Geometry check sheet. Reference: the model listing, model coordinates, mm. A direction names the side the tool comes from. Give positions to 0.01 mm unless a question says otherwise; leave off trailing zeros. Loops run counter-clockwise (first coordinate to the right, second up) from the corner with the lowest first, then second, coordinate; pieces in that order, holes last. Notation, with made-up numbers: (59.5, -20.75) -> (110.5, -20.75) arc R23 cw to (110.5, 15.25) -> close; hole circle Ø9 at (69, 53). An arc over 180 degrees is marked (long way). Answer as a JSON object with one key per item and string values.
from build123d import *

# Parameters (mm, degrees)
F1_DEPTH = 10
F2_R     = 3
F3_DEPTH = 10
F4_R     = 1.5
F5_DEPTH = 25
F6_R     = 3
F7_DEPTH = 5


with BuildPart() as f1:
    # F0 (on Right) → F1 (new body)
    with BuildSketch(Plane.YZ):
        Polygon((2.886751, 5), (-2.886751, 5), (-5.773503, 0), (-2.886751, -5), (2.886751, -5), (5.773503, 0), align=None)
    extrude(amount=F1_DEPTH)

    # F2 (on face) → F3 (join)
    with BuildSketch(Plane.YZ.offset(10)):
        Circle(F2_R)
    extrude(amount=F3_DEPTH)

    # F4 (on face) → F5 (cut)
    with BuildSketch(Plane(origin=(0, 0, 0), x_dir=(0, -1, 0), z_dir=(-1, 0, 0))):
        Circle(F4_R)
    extrude(amount=-F5_DEPTH, mode=Mode.SUBTRACT)

    # F6 (on face) → F7 (cut)
    with BuildSketch(Plane(origin=(0, 0, 0), x_dir=(0, -1, 0), z_dir=(-1, 0, 0))):
        Circle(F6_R)
    extrude(amount=-F7_DEPTH, mode=Mode.SUBTRACT)


solid = f1.part
1) Tool access check on faces 1 (the face through (15, -3, 0)), 2 (the face through (4.93, -4.35, -2.465)). Record the directions out of +Z, -Z, +X, -X, +Y, -Y that give a thin tool (end or side, any length) a straight path to the whole face; none if there is none.
Geometry check:
{"face 1": "+X", "face 2": "-Z, +X, -X, -Y"}
2) Section check D-D on x = 2. Record the cut outline in (y, z).
Geometry check:
{"outline": "(-5.77, 0) -> (-2.89, -5) -> (2.89, -5) -> (5.77, 0) -> (2.89, 5) -> (-2.89, 5) -> close; hole circle Ø6 at (0, 0)"}
3) Depth check by flat-ended pin: P1, Ø1.5, axis at y = 0, z = 2, coming from the -X side; P2, Ø5, axis at x = 15, z = 0, coming from the -Y side; P3, Ø1.5, axis at x = 2.5, y = -4, coming from the -Z side. Enter the tip coordinate at first touch or a pass-through.
Geometry check:
{"P1": "stops at x = 5", "P2": "stops at y = -3", "P3": "stops at z = -4.37"}
4) Material ranges on line 1 along Z through (x, y) = (3.5, 0); line 2 along Z through (x, y) = (14.5, 0); line 3 along X through (y, z) = (-4, -1.25), recorded low to high. Write a range as from..to.
Geometry check:
{"line 1": "z = -5..-3, 3..5", "line 2": "z = -3..-1.5, 1.5..3", "line 3": "x = 0..10"}
5) Section check B-B on x = 5.75. Record the cut outline in (y, z), plus the area to 3 significant figures.
Geometry check:
{"outline": "(-5.77, 0) -> (-2.89, -5) -> (2.89, -5) -> (5.77, 0) -> (2.89, 5) -> (-2.89, 5) -> close; hole circle Ø3 at (0, 0)", "area": "79.5 mm2"}
6) Section check C-C on z = -0.5. Record the cut outline in (x, y).
Geometry check:
{"outline": "(0, -5.48) -> (10, -5.48) -> (10, -2.96) -> (20, -2.96) -> (20, -1.41) -> (5, -1.41) -> (5, -2.96) -> (0, -2.96) -> close; (0, 2.96) -> (5, 2.96) -> (5, 1.41) -> (20, 1.41) -> (20, 2.96) -> (10, 2.96) -> (10, 5.48) -> (0, 5.48) -> close"}
7) Draft check along Y on faces 3 (the face through (5, -1.3, -1.3)), 4 (the face through (4.93, 4.35, 2.465)), 5 (the face through (4.93, -4.31, 2.535)), 6 (the face through (2, 3, 0)). Enter one of: pulls with the +Y half, pulls with the -Y half, needs draft (parallel to the pull), parting line crosses it, or undercut.
Geometry check:
{"face 3": "undercut", "face 4": "pulls with the +Y half", "face 5": "pulls with the -Y half", "face 6": "undercut"}
8) Section check A-A on y = 0. Record the cut outline in (x, z).
Geometry check:
{"outline": "(0, -5) -> (10, -5) -> (10, -3) -> (20, -3) -> (20, -1.5) -> (5, -1.5) -> (5, -3) -> (0, -3) -> close; (0, 3) -> (5, 3) -> (5, 1.5) -> (20, 1.5) -> (20, 3) -> (10, 3) -> (10, 5) -> (0, 5) -> close"}
